Input: part model. Units: mm. Frame: model coordinates. A direction names the side the tool comes from. Coordinates: 2 decimals unless noted, no trailing zeros. Loops run counter-clockwise (first coordinate to the right, second up) from the corner with the lowest first, then second, coordinate; pieces in that order, holes last.
Item 1: Section D-D on z = -189. Return loops of the section in (x, y).
Item 2: Section A-A on x = -81.28. Return loops of the section in (y, z) (3 decimals).
Item 3: Ray query, line 1 along Z through (x, y) = (-81.28, 14); line 2 along X through (y, z) = (16, -210); line 3 along Z through (x, y) = (-125, 409). Return the intervals inside material, ascending.
Item 4: Pull-direction query (Z, two-part tool) for faces 1 (the flat face through (-80, 228, 0)), 2 (the cylindrical face through (-63.7, 12.52, -244.62)), 3 (the cylindrical face through (-77.39, 357.76, -148.15)), 4 (the flat face through (-81, 388, -180.34)); classes: released by +Z, released by -Z, zero draft, split by the parting line, or undercut.
Item 5: Section C-C on y = 156.5. Return loops of the section in (x, z), and give its area (3 significant figures).
Item 6: Section B-B on z = -228. Return loops of the section in (x, y).
Item 7: Reachability of faces 5 (the flat face through (-80, 73.66, -193)), 6 (the cylindrical face through (-68.34, 445.62, -106.54)), 7 (the flat face through (-82, 25.4, -210)) from +Z, -Z, +X, -X, +Y, -Y: full face, straight path, thin tool, end or side. Return the list, or none.
Item 8: Contact query for flat-ended pins moving along their axis: P1, Ø4, axis at y = 377, z = -182, coming from the +X side; P2, Ø3, axis at x = -138.5, z = -200, coming from the +Y side; P3, Ø10, axis at x = -52.5, z = -207, coming from the -Y side. Output: stop coordinate, or through.
Autodesk Inventor part; units mm, degrees
ref_plane "YZ Plane" through (0, 0, 0) normal (1, 0, 0) x (0, 1, 0)
ref_plane "XZ Plane" through (0, 0, 0) normal (0, 1, 0) x (-1, 0, 0)
ref_plane "XY Plane" through (0, 0, 0) normal (0, 0, 1) x (1, 0, 0)
sketch "Sketch1" plane through (0, 0, 0) normal (0, 1, 0) x (-1, 0, 0)
  line L0 (0, 0) -> (162.56, 0)
  line L1 (162.56, 0) -> (162.56, -210.82)
  line L2 (81.28, -292.1) -> (81.28, -292.1)
  line L3 (0, -210.82) -> (0, 0)
  arc A0 (81.28, -292.1) -> (162.56, -210.82) centre (81.28, -210.82) ccw
  arc A1 (0, -210.82) -> (81.28, -292.1) centre (81.28, -210.82) ccw
  point P0 (162.56, -292.1)
  point P1 (0, -292.1)
  dimension "d0" = 292.1
  dimension "d1" = 162.56
  dimension "d2" = 81.28
extrude "Extrusion1" add sketch "Sketch1" along normal blind 73.66
sketch "Sketch2" plane through (0, 73.66, 0) normal (0, 1, 0) x (1, 0, 0)
  line L0 (-162.56, 0) -> (0, 0)
  line L1 (0, 0) -> (0, 210.82)
  line L2 (-162.56, 0) -> (0, 0)
  line L3 (0, 0) -> (0, 96.52)
  line L4 (0, 96.52) -> (-162.56, 96.52)
  line L5 (-162.56, 96.52) -> (-162.56, 0)
  dimension "d23" = 114.3
extrude "Extrusion2" add sketch "Sketch2" along normal blind 388.62
sketch "Sketch3" plane through (-162.56, 0, 0) normal (0, 0, 1) x (1, 0, 0)
  line L0 (162.56, 0) -> (0, 0)
  line L1 (162.56, 0) -> (162.56, 462.28)
  line L2 (0, 0) -> (162.56, 0)
  line L3 (162.56, 0) -> (162.56, 431.8)
  line L4 (132.08, 462.28) -> (30.48, 462.28)
  line L5 (0, 431.8) -> (0, 0)
  arc A0 (30.48, 462.28) -> (0, 431.8) centre (30.48, 431.8) ccw
  arc A1 (162.56, 431.8) -> (132.08, 462.28) centre (132.08, 431.8) ccw
  dimension "d8" = 30.48
extrude "Extrusion3" cut sketch "Sketch3" against normal blind 508 keep common part
sketch "Sketch4" plane through (0, 73.66, -96.52) normal (0, 0, -1) x (-1, 0, 0)
  line L0 (132.08, 388.62) -> (30.48, 388.62)
  circle A0 centre (81.28, 313.69) radius 59.69
  line L1 (0, -73.66) -> (162.56, -73.66)
  dimension "d12" = 119.38
  dimension "d22" = 387.35
extrude "Extrusion4" add sketch "Sketch4" along normal blind 20.32
sketch "Sketch5" plane through (-81.28, 387.35, -116.84) normal (0, 0, -1) x (-1, 0, 0)
  circle A0 centre (0, 0) radius 29.845
  point P0 (-81.28, -387.35)
  dimension "d15" = 59.69
extrude "Extrusion5" add sketch "Sketch5" along normal blind 63.5
sketch "Sketch6" plane through (0, 0, 0) normal (0, -1, 0) x (1, 0, 0)
  arc A0 (-162.56, -210.82) -> (0, -210.82) centre (-81.28, -210.82) ccw
  circle A1 centre (-81.28, -210.82) radius 38.1
  point P0 (0, 0)
  dimension "d18" = 76.2
extrude "Extrusion6" cut sketch "Sketch6" against normal blind 25.4
properties part number "Waist Link-lrg"
Results found:
1. outline: (-162.56, 0) - (-112.51, 0) - (-112.51, 25.4) - (-50.05, 25.4) - (-50.05, 0) - (0, 0) - (0, 73.66) - (-162.56, 73.66) - close
2. outline: (0, -292.1) - (73.66, -292.1) - (73.66, -96.52) - (327.66, -96.52) - (327.66, -116.84) - (357.505, -116.84) - (357.505, -180.34) - (417.195, -180.34) - (417.195, -116.84) - (447.04, -116.84) - (447.04, -96.52) - (462.28, -96.52) - (462.28, 0) - (0, 0) - (0, -172.72) - (25.4, -172.72) - (25.4, -248.92) - (0, -248.92) - close
3. line 1: z = -292.1 to -248.92, -172.72 to 0
3. line 2: x = -162.56 to -119.37, -43.19 to 0
3. line 3: z = -116.84 to 0
4. face 1: released by +Z
4. face 2: undercut
4. face 3: zero draft
4. face 4: released by -Z
5. outline: (-162.56, -96.52) - (0, -96.52) - (0, 0) - (-162.56, 0) - close
5. area: 15,700 mm2
6. outline: (-160.72, 0) - (-115.29, 0) - (-115.29, 25.4) - (-47.27, 25.4) - (-47.27, 0) - (-1.84, 0) - (-1.84, 73.66) - (-160.72, 73.66) - close
7. face 5: -Z, +X, -X
7. face 6: -Z
7. face 7: -Y
8. P1: stops at x = -52.9
8. P2: stops at y = 73.66
8. P3: stops at y = 25.4
